```python
from build123d import *

# Parameters (mm, degrees)
BASE_FLANGE1_DEPTH = 76
CUT_EXTRUDE1_REACH = 84.503
SKETCH2_R          = 1.640689261
SKETCH2_R_2        = 1.533997934
SKETCH2_R_3        = 2
CUT_EXTRUDE2_REACH = 88.104
SKETCH3_R          = 2


# Sheet-metal steps are written as plain solids
with BuildPart() as part:
    # Sketch1 → Base-Flange1 (new body)
    with BuildSketch(Plane(origin=(0, 0, 0), x_dir=(1, 0, 0), z_dir=(0, 1, 0))):
        with BuildLine():
            Line((19.325, -10), (-18.885, -10))
            ThreePointArc((-18.885, -10), (-19.196126984, -9.871126984), (-19.325, -9.56))
            Line((-19.325, -9.56), (-19.325, 9.56))
            ThreePointArc((-19.325, 9.56), (-19.196126984, 9.871126984), (-18.885, 10))
            Line((-18.885, 10), (19.325, 10))
            Line((19.325, 10), (19.325, 12))
            Line((19.325, 12), (-18.885, 12))
            ThreePointArc((-18.885, 12), (-20.610340546, 11.285340546), (-21.325, 9.56))
            Line((-21.325, 9.56), (-21.325, -9.56))
            ThreePointArc((-21.325, -9.56), (-20.610340546, -11.285340546), (-18.885, -12))
            Line((-18.885, -12), (19.325, -12))
            Line((19.325, -12), (19.325, -10))
        make_face()
    extrude(amount=BASE_FLANGE1_DEPTH)

    # Cut-Extrude1: up to this face of the body (flat: up to its plane)
    cut_extrude1_end = Plane(part.part.faces().sort_by_distance((0.22, 38, 12))[0])
    # Sketch2 → Cut-Extrude1 (cut, up to the picked face)
    with BuildSketch(Plane(origin=(0, 0, -12), x_dir=(-1, 0, 0), z_dir=(0, 0, -1)), mode=Mode.PRIVATE) as cut_extrude1_sk1:
        with Locations((-6.845, 67.2)):
            Circle(SKETCH2_R)
    cut_extrude1_tool1 = split(extrude(cut_extrude1_sk1.sketch, amount=-CUT_EXTRUDE1_REACH, mode=Mode.PRIVATE), bisect_by=cut_extrude1_end, keep=Keep.BOTH, mode=Mode.PRIVATE)
    # Sketch2 → Cut-Extrude1 (cut, up to the picked face)
    with BuildSketch(Plane(origin=(0, 0, -12), x_dir=(-1, 0, 0), z_dir=(0, 0, -1)), mode=Mode.PRIVATE) as cut_extrude1_sk2:
        with Locations((-6.845, 25.5)):
            Circle(SKETCH2_R_2)
    cut_extrude1_tool2 = split(extrude(cut_extrude1_sk2.sketch, amount=-CUT_EXTRUDE1_REACH, mode=Mode.PRIVATE), bisect_by=cut_extrude1_end, keep=Keep.BOTH, mode=Mode.PRIVATE)
    # Sketch2 → Cut-Extrude1 (cut, up to the picked face)
    with BuildSketch(Plane(origin=(0, 0, -12), x_dir=(-1, 0, 0), z_dir=(0, 0, -1)), mode=Mode.PRIVATE) as cut_extrude1_sk3:
        with Locations((-6.825, 48)):
            Circle(SKETCH2_R_3)
    cut_extrude1_tool3 = split(extrude(cut_extrude1_sk3.sketch, amount=-CUT_EXTRUDE1_REACH, mode=Mode.PRIVATE), bisect_by=cut_extrude1_end, keep=Keep.BOTH, mode=Mode.PRIVATE)
    # Sketch2 → Cut-Extrude1 (cut, up to the picked face)
    with BuildSketch(Plane(origin=(0, 0, -12), x_dir=(-1, 0, 0), z_dir=(0, 0, -1)), mode=Mode.PRIVATE) as cut_extrude1_sk4:
        with Locations((-15.325, 48)):
            Circle(SKETCH2_R_3)
    cut_extrude1_tool4 = split(extrude(cut_extrude1_sk4.sketch, amount=-CUT_EXTRUDE1_REACH, mode=Mode.PRIVATE), bisect_by=cut_extrude1_end, keep=Keep.BOTH, mode=Mode.PRIVATE)
    add(cut_extrude1_tool1.solids().sort_by(Axis((6.845, 67.2, -12), (0, 0, 1)))[0], mode=Mode.SUBTRACT)
    add(cut_extrude1_tool2.solids().sort_by(Axis((6.845, 25.5, -12), (0, 0, 1)))[0], mode=Mode.SUBTRACT)
    add(cut_extrude1_tool3.solids().sort_by(Axis((6.825, 48, -12), (0, 0, 1)))[0], mode=Mode.SUBTRACT)
    add(cut_extrude1_tool4.solids().sort_by(Axis((15.325, 48, -12), (0, 0, 1)))[0], mode=Mode.SUBTRACT)

    # Sketch3 → Cut-Extrude2 (cut, up to next)
    with BuildSketch(Plane(origin=(-19.325, 0, 0), x_dir=(0, 0, -1), z_dir=(1, 0, 0)), mode=Mode.PRIVATE) as cut_extrude2_sk1:
        with Locations((0, 68)):
            Circle(SKETCH3_R)
    cut_extrude2_tool1 = extrude(cut_extrude2_sk1.sketch, amount=-CUT_EXTRUDE2_REACH, mode=Mode.PRIVATE) & part.part
    # Sketch3 → Cut-Extrude2 (cut, up to next)
    with BuildSketch(Plane(origin=(-19.325, 0, 0), x_dir=(0, 0, -1), z_dir=(1, 0, 0)), mode=Mode.PRIVATE) as cut_extrude2_sk2:
        with Locations((0, 8)):
            Circle(SKETCH3_R)
    cut_extrude2_tool2 = extrude(cut_extrude2_sk2.sketch, amount=-CUT_EXTRUDE2_REACH, mode=Mode.PRIVATE) & part.part
    add(cut_extrude2_tool1.solids().sort_by_distance((-19.325, 68, 0))[0], mode=Mode.SUBTRACT)
    add(cut_extrude2_tool2.solids().sort_by_distance((-19.325, 8, 0))[0], mode=Mode.SUBTRACT)


solid = part.part
```
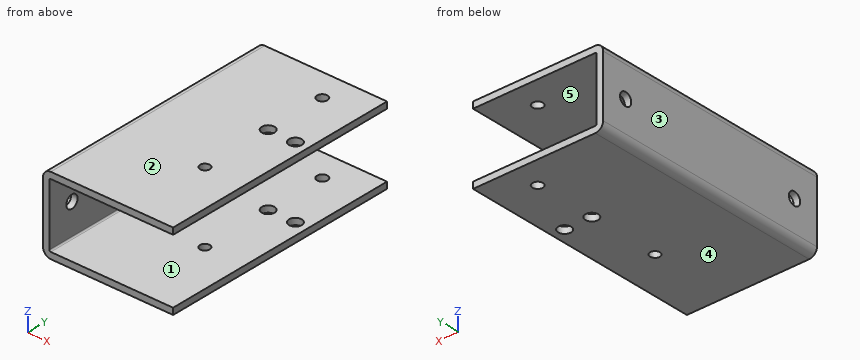
Input: part model. Units: mm. Frame: model coordinates. Face numbers are marked on the shaded views. A direction names the side the tool comes from. Coordinates: 2 decimals unless noted, no trailing zeros. Write each loop counter-clockwise with the first axis right and the second up, starting at its lowest first coordinate (ties: lowest second). Pieces come first, ordered by that corner, then holes. Notation, with made-up numbers: M -21,19 L 33,19 A16 ccw 33,50 Z; hole C 69.25,-37 d9. An arc over 180 degrees is marked long. Use one line per item in the form item = value.
Q1. Set-up query: the marked faces 1 and 2. Return all of +Z, -Z, +X, -X, +Y, -Y with unobstructed straight access to the full face (end or side cutting, diameter ignored); none if empty.
Answer below:
face_1 = +X, +Y, -Y
face_2 = +Z, +X, -X, +Y, -Y
Q2. Section C-C (x = 10). Return loops of the section in (y, z), plus the area to 3 significant figures.
Answer below:
outline = M 0,-12 L 76,-12 L 76,-10 L 0,-10 Z; M 0,10 L 76,10 L 76,12 L 0,12 Z
area = 304 mm²
Q3. Section A-A (z = 0). Return loops of the section in (x, y) (3 decimals), plus the area to 3 significant figures.
Answer below:
outline = M -21.325,0 L -19.325,0 L -19.325,6 L -21.325,6 Z; M -21.325,10 L -19.325,10 L -19.325,66 L -21.325,66 Z; M -21.325,70 L -19.325,70 L -19.325,76 L -21.325,76 Z
area = 136 mm²
Q4. Section D-D (y = 25.5). Return loops of the section in (x, z) (3 decimals).
Answer below:
outline = M -21.325,-9.56 A2.44 ccw -18.885,-12 L 5.311,-12 L 5.311,-10 L -18.885,-10 A0.44 cw -19.325,-9.56 L -19.325,9.56 A0.44 cw -18.885,10 L 5.311,10 L 5.311,12 L -18.885,12 A2.44 ccw -21.325,9.56 Z; M 8.379,-12 L 19.325,-12 L 19.325,-10 L 8.379,-10 Z; M 8.379,10 L 19.325,10 L 19.325,12 L 8.379,12 Z
Q5. Draft query along Z for the marked faces 3, 4 and 5. Return one class per face: released by +Z, released by -Z, zero draft, split by the parting line, or undercut.
Answer below:
face_3 = zero draft
face_4 = released by -Z
face_5 = undercut
Q6. Material intervals for probe 1 along Z at (x, y) = (-16, 65); probe 2 along X at (y, z) = (58, -2.5) (3 decimals); probe 3 along X at (y, z) = (32, 11) (3 decimals), sorted ascending. Write a range as from..to.
Answer below:
probe_1 = -12..-10, 10..12
probe_2 = -21.325..-19.325
probe_3 = -20.855..19.325
Q7. Section B-B (y = 8). Return loops of the section in (x, z) (3 decimals).
Answer below:
outline = M -21.325,-9.56 A2.44 ccw -18.885,-12 L 19.325,-12 L 19.325,-10 L -18.885,-10 A0.44 cw -19.325,-9.56 L -19.325,-2 L -21.325,-2 Z; M -21.325,2 L -19.325,2 L -19.325,9.56 A0.44 cw -18.885,10 L 19.325,10 L 19.325,12 L -18.885,12 A2.44 ccw -21.325,9.56 Z
Q8. First-contact query: pin 1 (9.5 mm diameter, centred on y = 30, z = -3, fed in from +X) (3 decimals). Flat tip, straight axial feed; report the tip coordinate or a pass-through.
Answer below:
pin_1 = -19.325
